from build123d import *

# Parameters (mm, degrees)
SKETCH1_R                = 3.875
BOSS_EXTRUDE1_DEPTH      = 9
BOSS_EXTRUDE1_DEPTH_BACK = 4
SKETCH2_R                = 5.4
BOSS_EXTRUDE2_DEPTH      = 9
SKETCH7_R                = 10
BOSS_EXTRUDE4_DEPTH      = 8
SKETCH8_R                = 2.25
CUT_EXTRUDE4_DEPTH       = 1
CUT_EXTRUDE4_DEPTH_BACK  = 14
CUT_EXTRUDE2_START       = -9
SKETCH3_R                = 1.375
CUT_EXTRUDE2_DEPTH       = 10
CIRPATTERN2_COUNT        = 4


with BuildPart() as part:
    # Sketch1 → Boss-Extrude1 (new body, two sides)
    with BuildSketch(Plane(origin=(0, 0, 0), x_dir=(1, 0, 0), z_dir=(0, 1, 0))) as boss_extrude1_sk:
        Circle(SKETCH1_R)
    extrude(amount=BOSS_EXTRUDE1_DEPTH)
    extrude(boss_extrude1_sk.sketch, amount=-BOSS_EXTRUDE1_DEPTH_BACK)

    # Sketch2 → Boss-Extrude2 (add)
    with BuildSketch(Plane(origin=(0, 0, 0), x_dir=(1, 0, 0), z_dir=(0, 1, 0))):
        Circle(SKETCH2_R)
    extrude(amount=BOSS_EXTRUDE2_DEPTH)

    # Sketch7 → Boss-Extrude4 (add)
    with BuildSketch(Plane(origin=(0, 9, 0), x_dir=(1, 0, 0), z_dir=(0, 1, 0))):
        Circle(SKETCH7_R)
    extrude(amount=-BOSS_EXTRUDE4_DEPTH)

    # Sketch8 → Cut-Extrude4 (cut, two sides)
    with BuildSketch(Plane.XZ.offset(4)) as cut_extrude4_sk:
        Circle(SKETCH8_R)
    extrude(amount=CUT_EXTRUDE4_DEPTH, mode=Mode.SUBTRACT)
    extrude(cut_extrude4_sk.sketch, amount=-CUT_EXTRUDE4_DEPTH_BACK, mode=Mode.SUBTRACT)

    # Sketch3 → Cut-Extrude2 (cut)
    with BuildSketch(Plane(origin=(0, 9, 0), x_dir=(1, 0, 0), z_dir=(0, 1, 0)).offset(CUT_EXTRUDE2_START)):
        with Locations((-7.75, 0)):
            Circle(SKETCH3_R)
    cut_extrude2 = extrude(amount=CUT_EXTRUDE2_DEPTH, mode=Mode.SUBTRACT)

    # CirPattern2: Cut-Extrude2 ×4 about axis
    cirpattern2_axis = Axis((0, 0, 0), (0, 1, 0))
    for i in range(1, CIRPATTERN2_COUNT):
        add(cut_extrude2.rotate(cirpattern2_axis, i * 360 / CIRPATTERN2_COUNT), mode=Mode.SUBTRACT)


solid = part.part
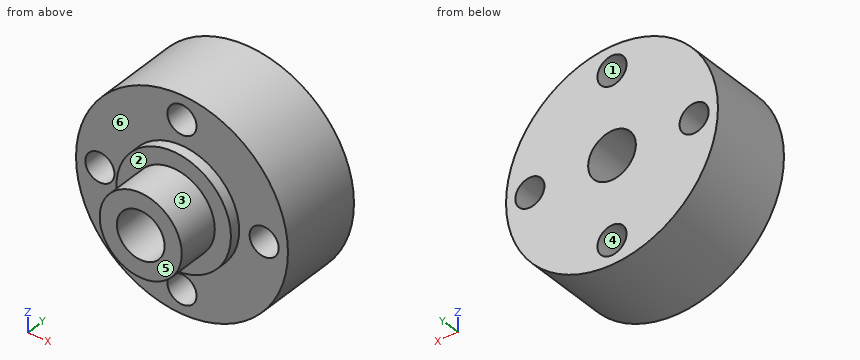
For this review, take the finished solid that the model builds, in its own axes (mm). Face numbers are marked on the shaded views. A direction names the side the tool comes from. Round coordinates to 2 decimals unless told otherwise and drop trailing zeros. Loops run counter-clockwise (first coordinate to the right, second up) from the corner with the lowest first, then second, coordinate; pieces in that order, holes last. Notation, with made-up numbers: (-38, 53) - (-21, 53) arc R14 ccw to (-21, 63) - close; hole circle Ø6 at (-23, -6). An arc over 180 degrees is marked (long way). One line per question, with ' | ' between items.
Q1. The part is to be moulded in two halves that separate along X. For the marked faces 1, 2, 3 and 4, say which applies: released by +X, released by -X, zero draft, split by the parting line, or undercut.
Taken from the geometry:
face 1: undercut | face 2: zero draft | face 3: split by the parting line | face 4: undercut
Q2. For line 1 along Y through (x, z) = (1.75, -6.75); line 2 along X through (y, z) = (-1.25, -0.5); line 3 along Z through (x, y) = (7.75, 5.5) (3 decimals), list the stretches that pass through material, from the lowest coordinate up. Write a range as [from, to].
Taken from the geometry:
line 1: y = [1, 9] | line 2: x = [-3.84, -2.19], [2.19, 3.84] | line 3: z = [-6.32, -1.375], [1.375, 6.32]
Q3. Tool access review of the marked faces 5 and 6: name each direction out of +Z, -Z, +X, -X, +Y, -Y from which nothing blocks a thin tool from reaching the whole face with its end or side.
Taken from the geometry:
face 5: +Z, -Z, +X, -X, -Y | face 6: -Y
Q4. Take a section at D-D (x = 7.5). Give the boundary of the cut face in (y, z), and give its area (3 significant figures).
Taken from the geometry:
outline: (1, -6.61) - (9, -6.61) - (9, -1.35) - (1, -1.35) - close; (1, 1.35) - (9, 1.35) - (9, 6.61) - (1, 6.61) - close | area: 84.2 mm²
Q5. Take a section at A-A (x = 0). Give the boundary of the cut face in (y, z) (3 decimals).
Taken from the geometry:
outline: (-4, -3.875) - (0, -3.875) - (0, -5.4) - (1, -5.4) - (1, -6.375) - (9, -6.375) - (9, -2.25) - (-4, -2.25) - close; (-4, 2.25) - (9, 2.25) - (9, 6.375) - (1, 6.375) - (1, 5.4) - (0, 5.4) - (0, 3.875) - (-4, 3.875) - close; (1, -10) - (9, -10) - (9, -9.125) - (1, -9.125) - close; (1, 9.125) - (9, 9.125) - (9, 10) - (1, 10) - close
Q6. For pin 1 (4.5 mm diameter, centred on x = 0, z = -7.75, fed in from -Y); pin 2 (3 mm diameter, centred on y = -2.5, z = 7, fed in from +X); pin 3 (5 mm diameter, centred on y = -2, z = 0, fed in from -X); pin 4 (4 mm diameter, centred on x = -2.5, y = 0.5, fed in from +Z), all flat-tipped, find the tip position at first contact; note any pin that passes through.
Taken from the geometry:
pin 1: stops at y = 1 | pin 2: passes through | pin 3: stops at x = -5.4 | pin 4: stops at z = 9.98
Q7. Take a section at B-B (y = 4). Give the boundary of the cut face in (x, z) (3 decimals), and give its area (3 significant figures).
Taken from the geometry:
outline: circle Ø20 at (0, 0); hole circle Ø2.75 at (-7.75, 0); hole circle Ø4.5 at (0, 0); hole circle Ø2.75 at (0, -7.75); hole circle Ø2.75 at (0, 7.75); hole circle Ø2.75 at (7.75, 0) | area: 274 mm²
Q8. Take a section at C-C (z = -8.25). Give the boundary of the cut face in (x, y), and give its area (3 significant figures).
Taken from the geometry:
outline: (-5.65, 1) - (-1.28, 1) - (-1.28, 9) - (-5.65, 9) - close; (1.28, 1) - (5.65, 1) - (5.65, 9) - (1.28, 9) - close | area: 69.9 mm²
